Autodesk Inventor part; units mm, degrees
ref_plane "YZ Plane" through (0, 0, 0) normal (1, 0, 0) x (0, 1, 0)
ref_plane "XZ Plane" through (0, 0, 0) normal (0, 1, 0) x (-1, 0, 0)
ref_plane "XY Plane" through (0, 0, 0) normal (0, 0, 1) x (1, 0, 0)
sketch "maiin" plane through (0, 0, 0) normal (0, 0, 1) x (1, 0, 0)
  circle A0 centre (114.3234, 350.4213) radius 2.1844
  circle A1 centre (127.0234, 350.4213) radius 2.1844
  line L0 (86.4201, 300.7833) -> (108.4755, 352.8962)
  arc A2 (86.4201, 300.7833) -> (85.4157, 295.8335) centre (98.1157, 295.8335) ccw
  line L1 (209.5734, 102.7713) -> (133.0946, 352.2822)
  line L2 (209.5734, 96.4213) -> (209.5734, 102.7713)
  circle A3 centre (203.2234, 96.4213) radius 2.1844
  arc A4 (209.45, 95.176) -> (209.5734, 96.4213) centre (203.2234, 96.4213) ccw
  line L3 (196.75, 31.676) -> (209.45, 95.176)
  circle A5 centre (190.5234, 32.9213) radius 2.1844
  line L4 (85.4157, 295.8335) -> (85.4157, 3.6912)
  circle A6 centre (127.0234, -17.8787) radius 2.1844
  circle A7 centre (114.3234, -17.8787) radius 2.1844
  arc A8 (127.0234, -24.2287) -> (130.9902, -22.8372) centre (127.0234, -17.8787) ccw
  arc A9 (110.2871, -22.7809) -> (114.3234, -24.2287) centre (114.3234, -17.8787) ccw
  arc A10 (194.4902, 27.9628) -> (196.75, 31.676) centre (190.5234, 32.9213) ccw
  arc A11 (85.4157, 3.6912) -> (90.0433, -6.1132) centre (98.1157, 3.6912) ccw
  line L5 (130.9902, -22.8372) -> (194.4902, 27.9628)
  line L6 (110.2871, -22.7809) -> (90.0433, -6.1132)
  line L7 (114.3234, -24.2287) -> (127.0234, -24.2287)
  arc A12 (114.3234, 356.7713) -> (108.4755, 352.8962) centre (114.3234, 350.4213) ccw
  line L8 (127.0234, 356.7713) -> (114.3234, 356.7713)
  arc A13 (133.0946, 352.2822) -> (127.0234, 356.7713) centre (127.0234, 350.4213) ccw
  point P0 (137.6055, 139.9011)
  point P1 (110.8157, 355.7146)
  dimension "d0" = 12.7
  dimension "d1" = 12.7
  dimension "d2" = 25.4
sketch "Sketch1" plane through (0, 0, 0) normal (1, 0, 0) x (0, 1, 0)
  circle A0 centre (-12.7, 0) radius 2.1844
  circle A1 centre (0, 0) radius 2.1844
  line L0 (-40.6033, -49.6379) -> (-18.5478, 2.4749)
  arc A2 (-40.6033, -49.6379) -> (-41.6076, -54.5878) centre (-28.9076, -54.5878) ccw
  line L1 (82.55, -247.65) -> (6.0712, 1.8609)
  line L2 (82.55, -254) -> (82.55, -247.65)
  circle A3 centre (76.2, -254) radius 2.1844
  arc A4 (82.4267, -255.2453) -> (82.55, -254) centre (76.2, -254) ccw
  line L3 (69.7267, -318.7453) -> (82.4267, -255.2453)
  circle A5 centre (63.5, -317.5) radius 2.1844
  line L4 (-41.6076, -54.5878) -> (-41.6076, -346.7301)
  circle A6 centre (0, -368.3) radius 2.1844
  circle A7 centre (-12.7, -368.3) radius 2.1844
  arc A8 (0, -374.65) -> (3.9668, -373.2585) centre (0, -368.3) ccw
  arc A9 (-16.7362, -373.2022) -> (-12.7, -374.65) centre (-12.7, -368.3) ccw
  arc A10 (67.4668, -322.4585) -> (69.7267, -318.7453) centre (63.5, -317.5) ccw
  arc A11 (-41.6076, -346.7301) -> (-36.98, -356.5344) centre (-28.9076, -346.7301) ccw
  line L5 (3.9668, -373.2585) -> (67.4668, -322.4585)
  line L6 (-16.7362, -373.2022) -> (-36.98, -356.5344)
  line L7 (-12.7, -374.65) -> (0, -374.65)
  arc A12 (-12.7, 6.35) -> (-18.5478, 2.4749) centre (-12.7, 0) ccw
  line L8 (0, 6.35) -> (-12.7, 6.35)
  arc A13 (6.0712, 1.8609) -> (0, 6.35) centre (0, 0) ccw
extrude "Extrusion1" add sketch "Sketch1" along normal blind 1.5875
properties part number "skirt" material "Acetal Resin, White"
Geometry check sheet. Reference: the model listing, model coordinates, mm. Coordinates: 2 decimals unless noted, no trailing zeros. Loops run counter-clockwise (first coordinate to the right, second up) from the corner with the lowest first, then second, coordinate; pieces in that order, holes last. Notation, with made-up numbers: (-16, 24.5) -> (29, 24.5) arc R35 cw to (29, 59.5) -> close; hole circle Ø7 at (15.5, 30). An arc over 180 degrees is marked (long way). Put each result on its own line as item: value.
1) Thickness scan on line 1 (Z direction, x = 0.75, y = -12.7); line 2 (Y direction, x = 1.1, z = -368.3). Record the ranges inside material, lowest first.
Result set:
line 1: z = -374.65 to -370.48, -366.12 to -2.18, 2.18 to 6.35
line 2: y = -22.69 to -14.88, -10.52 to -2.18, 2.18 to 10.16
2) Cross-section at A-A on x = 0.45. Record the boundary of the cut face in (y, z), plus the area to 3 significant figures.
Result set:
outline: (-41.61, -346.73) arc R12.7 ccw to (-36.98, -356.53) -> (-16.74, -373.2) arc R6.35 ccw to (-12.7, -374.65) -> (0, -374.65) arc R6.35 ccw to (3.97, -373.26) -> (67.47, -322.46) arc R6.35 ccw to (69.73, -318.75) -> (82.43, -255.25) arc R6.35 ccw to (82.55, -254) -> (82.55, -247.65) -> (6.07, 1.86) arc R6.35 ccw to (0, 6.35) -> (-12.7, 6.35) arc R6.35 ccw to (-18.55, 2.47) -> (-40.6, -49.64) arc R12.7 ccw to (-41.61, -54.59) -> close; hole circle Ø4.37 at (-12.7, -368.3); hole circle Ø4.37 at (-12.7, 0); hole circle Ø4.37 at (0, -368.3); hole circle Ø4.37 at (0, 0); hole circle Ø4.37 at (63.5, -317.5); hole circle Ø4.37 at (76.2, -254)
area: 33,300 mm^2
3) Cross-section at C-C on y = -24. Record the boundary of the cut face in (x, z).
Result set:
outline: (0, -367.22) -> (1.59, -367.22) -> (1.59, -10.41) -> (0, -10.41) -> close
4) Cross-section at B-B on y = 45. Record the boundary of the cut face in (x, z).
Result set:
outline: (0, -340.43) -> (1.59, -340.43) -> (1.59, -125.14) -> (0, -125.14) -> close
